Work out the finished part from the listing and answer in its coordinate system (mm). A direction names the side the tool comes from. Round coordinates to 2 decimals unless told otherwise and drop trailing zeros. Write item = value, one per line. Start each with the question number.
from build123d import *

# Parameters (mm, degrees)
CROQUIS1_W                                           = 12
CROQUIS1_H                                           = 500
SALIENTE_EXTRUIR1_DEPTH                              = 8
CORTAR_EXTRUIR1_DEPTH                                = 501.05240509
CORTAR_EXTRUIR2_DEPTH                                = 501.05240509
CORTAR_EXTRUIR3_DEPTH                                = 501.05240509
CORTAR_EXTRUIR4_DEPTH                                = 501.05240509
CORTAR_EXTRUIR5_DEPTH                                = 501.05240509
CORTAR_EXTRUIR6_DEPTH                                = 501.05240509
CORTAR_EXTRUIR7_DEPTH                                = 501.05240509
REFRENTADO_PARA_TORNILLO_CON_CABEZA_HEXA_D           = 3.5
REFRENTADO_PARA_TORNILLO_CON_CABEZA_HEXA_CBORE_D     = 6
REFRENTADO_PARA_TORNILLO_CON_CABEZA_HEXA_CBORE_DEPTH = 4.5
CHAFL_N1_SIZE                                        = 0.4
CHAFL_N2_SIZE                                        = 0.034056407
CHAFL_N2_SIZE_2                                      = 0.03688403
CHAFL_N3_SIZE                                        = 0.091173812
CHAFL_N3_SIZE_2                                      = 0.105000846
CROQUIS11_W                                          = 21.39366532
CROQUIS11_H                                          = 19.512682309
CORTAR_EXTRUIR8_DEPTH                                = 180


with BuildPart() as part:
    # Croquis1 → Saliente-Extruir1 (new body)
    with BuildSketch(Plane(origin=(0, 4.050658692, 0), x_dir=(1, 0, 0), z_dir=(0, 1, 0))):
        Rectangle(CROQUIS1_W, CROQUIS1_H)
    extrude(amount=-SALIENTE_EXTRUIR1_DEPTH)

    # Croquis2 → Cortar-Extruir1 (cut, through all)
    with BuildSketch(Plane(origin=(0, 0, -250), x_dir=(-1, 0, 0), z_dir=(0, 0, -1))):
        with BuildLine():
            Line((1.35, -3.949341308), (1.85, -3.949341308))
            ThreePointArc((1.85, -3.949341308), (1.6, -3.849341308), (1.35, -3.949341308))
        make_face()
    extrude(amount=-CORTAR_EXTRUIR1_DEPTH, mode=Mode.SUBTRACT)

    # Croquis3 → Cortar-Extruir2 (cut, through all)
    with BuildSketch(Plane(origin=(0, 0, -250), x_dir=(-1, 0, 0), z_dir=(0, 0, -1))):
        with BuildLine():
            Line((-6, 2.100658692), (-6, 1.200658692))
            Line((-6, 1.200658692), (-5.2, 1.200658692))
            ThreePointArc((-5.2, 1.200658692), (-4.75, 1.650658692), (-5.2, 2.100658692))
            Line((-5.2, 2.100658692), (-6, 2.100658692))
        make_face()
    extrude(amount=-CORTAR_EXTRUIR2_DEPTH, mode=Mode.SUBTRACT)

    # Croquis4 → Cortar-Extruir3 (cut, through all)
    with BuildSketch(Plane(origin=(0, 0, -250), x_dir=(-1, 0, 0), z_dir=(0, 0, -1))):
        with BuildLine():
            Line((-5.622557264, 1.200658692), (-6, 1.200658692))
            Line((-6, 1.200658692), (-6, 0.689297919))
            ThreePointArc((-6, 0.689297919), (-5.684900038, 0.851696449), (-5.622557264, 1.200658692))
        make_face()
    extrude(amount=-CORTAR_EXTRUIR3_DEPTH, mode=Mode.SUBTRACT)

    # Croquis5 → Cortar-Extruir4 (cut, through all)
    with BuildSketch(Plane(origin=(0, 0, -250), x_dir=(-1, 0, 0), z_dir=(0, 0, -1))):
        with BuildLine():
            Line((-6, 2.612019466), (-6, 2.100658692))
            Line((-6, 2.100658692), (-5.622557264, 2.100658692))
            ThreePointArc((-5.622557264, 2.100658692), (-5.684900038, 2.449620935), (-6, 2.612019466))
        make_face()
    extrude(amount=-CORTAR_EXTRUIR4_DEPTH, mode=Mode.SUBTRACT)

    # Croquis6 → Cortar-Extruir5 (cut, through all)
    with BuildSketch(Plane(origin=(0, 0, -250), x_dir=(-1, 0, 0), z_dir=(0, 0, -1))):
        with BuildLine():
            Line((6, 1.200658692), (6, 2.100658692))
            Line((6, 2.100658692), (5.2, 2.100658692))
            ThreePointArc((5.2, 2.100658692), (4.75, 1.650658692), (5.2, 1.200658692))
            Line((5.2, 1.200658692), (6, 1.200658692))
        make_face()
    extrude(amount=-CORTAR_EXTRUIR5_DEPTH, mode=Mode.SUBTRACT)

    # Croquis7 → Cortar-Extruir6 (cut, through all)
    with BuildSketch(Plane(origin=(0, 0, -250), x_dir=(-1, 0, 0), z_dir=(0, 0, -1))):
        with BuildLine():
            Line((5.622557264, 2.100658692), (6, 2.100658692))
            Line((6, 2.100658692), (6, 2.612019466))
            ThreePointArc((6, 2.612019466), (5.684900038, 2.449620935), (5.622557264, 2.100658692))
        make_face()
    extrude(amount=-CORTAR_EXTRUIR6_DEPTH, mode=Mode.SUBTRACT)

    # Croquis8 → Cortar-Extruir7 (cut, through all)
    with BuildSketch(Plane(origin=(0, 0, -250), x_dir=(-1, 0, 0), z_dir=(0, 0, -1))):
        with BuildLine():
            Line((6, 0.689297919), (6, 1.200658692))
            Line((6, 1.200658692), (5.622557264, 1.200658692))
            ThreePointArc((5.622557264, 1.200658692), (5.684900038, 0.851696449), (6, 0.689297919))
        make_face()
    extrude(amount=-CORTAR_EXTRUIR7_DEPTH, mode=Mode.SUBTRACT)

    # Refrentado para tornillo con cabeza hexagonal de M31 (through all)
    with Locations(Plane(origin=(0, 4.050658692, 0), x_dir=(1, 0, 0), z_dir=(0, 1, 0))):
        with Locations((0, -240), (0, -215), (0, -190), (0, -165), (0, -140), (0, -115), (0, -90), (0, -65), (0, -40), (0, -15), (0, 10), (0, 35), (0, 60), (0, 85), (0, 110), (0, 135), (0, 160), (0, 185), (0, 210), (0, 235)):
            CounterBoreHole(REFRENTADO_PARA_TORNILLO_CON_CABEZA_HEXA_D / 2, REFRENTADO_PARA_TORNILLO_CON_CABEZA_HEXA_CBORE_D / 2, REFRENTADO_PARA_TORNILLO_CON_CABEZA_HEXA_CBORE_DEPTH)

    # Chaflán1
    chafl_n1_edges = [part.edges().sort_by_distance(p)[0] for p in [
        (-6, -3.949341308, 0),
        (6, -3.949341308, 0),
        (-6, 4.050658692, 0),
        (6, 4.050658692, 0),
    ]]
    chamfer(chafl_n1_edges, length=CHAFL_N1_SIZE)

    # Chaflán2
    # the kernel refuses this chamfer: 0.03688403, 0.034056407 mm, written as the material it takes off along each edge
    with BuildSketch(Plane(origin=(6, 0.689297919, -250.100435582), x_dir=(-0.9978479381588691, 0.06557051404475742, 0), z_dir=(0, 0, 1))) as chafl_n2_piece_1:
        with BuildLine():
            Line((0.03902449, 0), (-CHAFL_N2_SIZE * 0.0655705141026, CHAFL_N2_SIZE * 0.997847939043))
            Line((-CHAFL_N2_SIZE * 0.0655705141026, CHAFL_N2_SIZE * 0.997847939043), (0, 0))
            ThreePointArc((0, 0), (0.020082989, 0.000475786), (0.03902449, 0))
        make_face()
    extrude(amount=500.200871164, mode=Mode.SUBTRACT)
    with BuildSketch(Plane(origin=(6, 2.612019466, -250.094971685), x_dir=(0, 1, 0), z_dir=(0, 0, 1))) as chafl_n2_piece_2:
        with BuildLine():
            Line((CHAFL_N2_SIZE_2 * 0.999999990825, 0), (-0.002179894, 0.035512658))
            ThreePointArc((-0.002179894, 0.035512658), (-0.000727719, 0.018309495), (0, 0))
            Line((0, 0), (CHAFL_N2_SIZE_2 * 0.999999990825, 0))
        make_face()
    extrude(amount=500.189943371, mode=Mode.SUBTRACT)
    with BuildSketch(Plane(origin=(-6, 2.612019466, -250.100435582), x_dir=(0, 1, 0), z_dir=(0, 0, 1))) as chafl_n2_piece_3:
        with BuildLine():
            Line((CHAFL_N2_SIZE, 0), (-0.002558856, -0.038940507))
            ThreePointArc((-0.002558856, -0.038940507), (-0.00084209, -0.020070966), (0, 0))
            Line((0, 0), (CHAFL_N2_SIZE, 0))
        make_face()
    extrude(amount=500.200871164, mode=Mode.SUBTRACT)
    with BuildSketch(Plane(origin=(-6, 0.689297919, -250.094971685), x_dir=(0.9981213351064977, 0.061268265890444186, 0), z_dir=(0, 0, 1))) as chafl_n2_piece_4:
        with BuildLine():
            Line((0.0355795, 0), (-CHAFL_N2_SIZE_2 * 0.0612682653281, -CHAFL_N2_SIZE_2 * 0.998121325949))
            Line((-CHAFL_N2_SIZE_2 * 0.0612682653281, -CHAFL_N2_SIZE_2 * 0.998121325949), (0, 0))
            ThreePointArc((0, 0), (0.018319684, -0.000395439), (0.0355795, 0))
        make_face()
    extrude(amount=500.189943371, mode=Mode.SUBTRACT)

    # Chaflán3
    # the kernel refuses this chamfer: 0.105000846, 0.091173812 mm, written as the material it takes off along each edge
    with BuildSketch(Plane(origin=(5.622557264, 1.200658692, -250.318147751), x_dir=(-0.1263625484615496, -0.991984126055605, 0), z_dir=(0, 0, 1)), Plane(origin=(-5.622557264, 2.100658692, -250.318147751), x_dir=(0.12636254846156672, 0.9919841260556028, 0), z_dir=(0, 0, 1))) as chafl_n3_piece_1:
        with BuildLine():
            Line((0.123959197, 0), (CHAFL_N3_SIZE * 0.126362548546, -CHAFL_N3_SIZE * 0.99198412672))
            Line((CHAFL_N3_SIZE * 0.126362548546, -CHAFL_N3_SIZE * 0.99198412672), (0, 0))
            ThreePointArc((0, 0), (0.063641461, -0.004827559), (0.123959197, 0))
        make_face()
    extrude(amount=500.636295502, mode=Mode.SUBTRACT)
    with BuildSketch(Plane(origin=(5.622557264, 2.100658692, -250.269677179), x_dir=(-1, 0, 0), z_dir=(0, 0, 1)), Plane(origin=(-5.622557264, 1.200658692, -250.269677179), x_dir=(1, 0, 0), z_dir=(0, 0, 1))) as chafl_n3_piece_2:
        with BuildLine():
            Line((CHAFL_N3_SIZE_2, 0), (0.015616157, -0.098323158))
            ThreePointArc((0.015616157, -0.098323158), (0.011085216, -0.04998658), (0, 0))
            Line((0, 0), (CHAFL_N3_SIZE_2, 0))
        make_face()
    extrude(amount=500.539354358, mode=Mode.SUBTRACT)

    # Croquis11 → Cortar-Extruir8 (cut)
    with BuildSketch(Plane(origin=(0, 0, -250), x_dir=(-1, 0, 0), z_dir=(0, 0, -1))):
        with Locations((-0.979177693, 1.955889883)):
            Rectangle(CROQUIS11_W, CROQUIS11_H)
    extrude(amount=-CORTAR_EXTRUIR8_DEPTH, mode=Mode.SUBTRACT)


solid = part.part
1. Which of the six approach directions +Z, -Z, +X, -X, +Y, -Y give full straight-line access (tool end or side, diameter ignored) to faces 1 (the face through (-0.65, 1.83, 67.93)), 2 (the face through (0, 0, 250))?
2. For a pull along Z with two mould halves and no side action, classify faces 3 (the face through (2, -3.949, 88)), 4 (the face through (0, 0, -70)), 5 (the face through (-0.65, 1.83, 17.93)) as released by +Z, released by -Z, zero draft, split by the parting line, or undercut.
3. Each of these flat-tipped pins is pushed along its axis until it touches: pin 1 (3 mm diameter, centred on x = 0, z = 215, fed in from +Y); pin 2 (4 mm diameter, centred on x = 0, z = 15, fed in from +Y). Where does it stop, or does it pass through?
4. Consider line 1 (X direction, y = -3.2, z = 140); line 2 (Y direction, x = -1.75, z = 75); line 3 (X direction, y = 1.5, z = -43). Determine where each line is inside the solid, lowest interval first.
Answer key:
q1.face_1 = +Y
q1.face_2 = +Z, +X, -X, +Y, -Y
q2.face_3 = zero draft
q2.face_4 = released by -Z
q2.face_5 = undercut
q3.pin_1 = through
q3.pin_2 = -0.45
q4.line_1 = -6 to -1.75, 1.75 to 6
q4.line_2 = -3.88 to 4.05
q4.line_3 = -4.78 to 4.78
